CAD build for the part. Positions are in the model's coordinates, mm. A direction names the side the tool comes from. Round coordinates to 2 decimals unless told otherwise and drop trailing zeros. Loops run counter-clockwise (first coordinate to the right, second up) from the corner with the lowest first, then second, coordinate; pieces in that order, holes last.
```python
from build123d import *

# Parameters (mm, degrees)
BOSS_EXTRUDE1_DEPTH = 50
SKETCH3_W           = 3.3
SKETCH3_H           = 1
BOSS_EXTRUDE2_DEPTH = 13
BOSS_EXTRUDE3_DEPTH = 57
CHAMFER1_START      = -14
CHAMFER1_OUTLINE_W  = 52
CHAMFER1_OUTLINE_H  = 13
CHAMFER1_DEPTH      = 3.182909169
CHAMFER2_SIZE       = 3


with BuildPart() as part:
    # Sketch2 → Boss-Extrude1 (new body)
    with BuildSketch(Plane(origin=(0, 0, 0), x_dir=(1, 0, 0), z_dir=(0, 1, 0))):
        Polygon((-1.7, -2), (-1.7, -15), (-5.7, -15), (-5.7, -2), (-9, -2), (-9, -15), (-13, -15), (-13, 2.680601608), align=None)
    extrude(amount=BOSS_EXTRUDE1_DEPTH)

    # Sketch3 → Boss-Extrude2 (add)
    with BuildSketch(Plane.XY.offset(2)):
        with Locations((-7.35, 0.5)):
            Rectangle(SKETCH3_W, SKETCH3_H)
    extrude(amount=BOSS_EXTRUDE2_DEPTH)

    # Sketch5 → Boss-Extrude3 (add)
    with BuildSketch(Plane.XY.offset(15)):
        Polygon((-13, 0), (-1.7, 0), (-1.7, 14), (-5.7, 14), (-5.7, 1), (-9, 1), (-9, 14), (-13, 14), align=None)
    extrude(amount=BOSS_EXTRUDE3_DEPTH)

    # Mirror1: part across plane


with BuildPart() as part_1:
    add(part.part)
    add(part.part.mirror(Plane(origin=(-0.956063716, 0, 2.308147732), x_dir=(0.9238798691632129, 0, 0.38268261961443256), z_dir=(0.3826826196144326, 0, -0.9238798691632131))))

    # Chamfer1: read off the stored shape, not the designer's step
    # Chamfer1 outline → Chamfer1 (cut)
    with BuildSketch(Plane(origin=(0, 0, 0), x_dir=(0, 1, 0), z_dir=(0.9238798691632129, 0, 0.38268261961443295)).offset(CHAMFER1_START)):
        with Locations((25, 2.5)):
            Rectangle(CHAMFER1_OUTLINE_W, CHAMFER1_OUTLINE_H)
    extrude(amount=CHAMFER1_DEPTH, mode=Mode.SUBTRACT)

    # Chamfer2
    chamfer2_edges = [part_1.edges().sort_by_distance(p)[0] for p in [
        (-13, 32, 15),
        (-13, 14, 43.5),
        (-0.497948704, 32, -15.182696898),
        (19.654559103, 14, -35.335275619),
    ]]
    chamfer(chamfer2_edges, length=CHAMFER2_SIZE)


solid = part_1.part
```
Item 1: Probe line 1 (X direction, y = 6.5, z = 65.5); line 2 (Y direction, x = -5.5, z = 38.5); line 3 (X direction, y = 9, z = -12). List the from-to ranges inside material, lowest first.
Answers follow:
line 1: x = -13 to -9, -5.7 to -1.7
line 2: y = 0 to 14
line 3: x = -3.68 to 1.98, 6.64 to 12.3
Item 2: Cut at B-B, the plane z = 23.5. Give the cut face in (x, y), plus the area to 3 significant figures.
Answers follow:
outline: (-13, 0) - (-1.7, 0) - (-1.7, 14) - (-5.7, 14) - (-5.7, 1) - (-9, 1) - (-9, 14) - (-10, 14) - (-13, 11) - close
area: 111 mm2
Item 3: Two-plate mould, pull along Z, no slides. Class faces 4 (the flat face through (8.874, 9.51, -14.231)), 5 (the flat face through (-4, 32, 15)), 6 (the flat face through (6.541, 8.824, -16.565)), 7 (the flat face through (22, 14, -33)): released by +Z, released by -Z, zero draft, split by the parting line, or undercut.
Answers follow:
face 4: undercut
face 5: released by +Z
face 6: undercut
face 7: zero draft
Item 4: Cut at A-A, the plane y = 39. Give the cut face in (x, z).
Answers follow:
outline: (-13, 3.12) - (-8.9, -6.78) - (-2.62, -13.06) - (1.62, -13.06) - (2.33, -12.35) - (-6.86, -3.16) - (-4.53, -0.83) - (4.66, -10.02) - (7.49, -7.19) - (-1.7, 2) - (-1.7, 15) - (-5.7, 15) - (-5.7, 2) - (-9, 2) - (-9, 15) - (-10, 15) - (-13, 12) - close
Item 5: Cut at C-C, the plane x = 27. Give the cut face in (y, z), plus the area to 3 significant figures.
Answers follow:
outline: (0, -42.68) - (11, -42.68) - (14, -38.44) - (14, -37.02) - (1, -37.02) - (1, -32.36) - (14, -32.36) - (14, -26.7) - (0, -26.7) - close
area: 157 mm2
Item 6: Flat gauge pins, fed straight in: P1, Ø5, axis at y = 7.5, z = 12, coming from the +X side; P2, Ø1.1, axis at x = -9.5, y = 37, coming from the +Z side; P3, Ø2, axis at x = 0.5, y = 27, coming from the -Z side. Where does each tip first touch, or does it go through?
Answers follow:
P1: stops at x = -1.7
P2: stops at z = 15
P3: stops at z = -13.06
Item 7: 3-axis set-ups, long thin cutter, end or side, ignore diameter. For faces 1 (the flat face through (-4, 14, 43)), 2 (the flat face through (19, 1, -26)), 3 (the flat face through (6.058, 32.252, -8.626)): which of +Z, -Z, +X, -X, +Y, -Y reach the whole face in a straight line?
Answers follow:
face 1: +Z, +X, -X, +Y
face 2: +Y
face 3: -Z, +X, +Y
